from build123d import *

# Parameters (mm, degrees)
SKETCH1_W           = 216
SKETCH1_H           = 166
SKETCH1_W_2         = 40
SKETCH1_H_2         = 3
SKETCH1_W_3         = 3
SKETCH1_H_3         = 30
BOSS_EXTRUDE1_DEPTH = 3


with BuildPart() as part:
    # Sketch1 → Boss-Extrude1 (new body)
    with BuildSketch(Plane.XY):
        Rectangle(SKETCH1_W, SKETCH1_H)
        with Locations((-80, 76.5)):
            Rectangle(SKETCH1_W_2, SKETCH1_H_2, mode=Mode.SUBTRACT)
        with Locations((80, 76.5)):
            Rectangle(SKETCH1_W_2, SKETCH1_H_2, mode=Mode.SUBTRACT)
        with Locations((101.5, 30)):
            Rectangle(SKETCH1_W_3, SKETCH1_H_3, mode=Mode.SUBTRACT)
        with Locations((80, -76.5)):
            Rectangle(SKETCH1_W_2, SKETCH1_H_2, mode=Mode.SUBTRACT)
        with Locations((-101.5, 30)):
            Rectangle(SKETCH1_W_3, SKETCH1_H_3, mode=Mode.SUBTRACT)
        with Locations((0, 76.5)):
            Rectangle(SKETCH1_W_2, SKETCH1_H_2, mode=Mode.SUBTRACT)
        with Locations((101.5, -30)):
            Rectangle(SKETCH1_W_3, SKETCH1_H_3, mode=Mode.SUBTRACT)
        with Locations((0, -76.5)):
            Rectangle(SKETCH1_W_2, SKETCH1_H_2, mode=Mode.SUBTRACT)
        with Locations((-80, -76.5)):
            Rectangle(SKETCH1_W_2, SKETCH1_H_2, mode=Mode.SUBTRACT)
        with Locations((-101.5, -30)):
            Rectangle(SKETCH1_W_3, SKETCH1_H_3, mode=Mode.SUBTRACT)
    extrude(amount=BOSS_EXTRUDE1_DEPTH)


solid = part.part
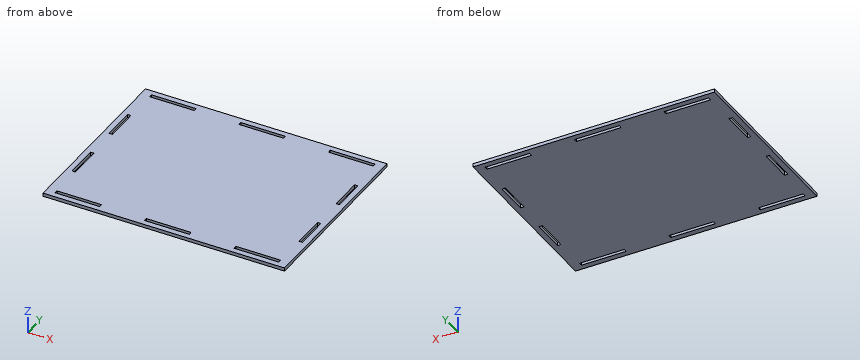
Can you work these out from the model? Positions are in its coordinate system, mm. Round coordinates to 2 decimals unless told otherwise and drop trailing zeros. Loops run counter-clockwise (first coordinate to the right, second up) from the corner with the lowest first, then second, coordinate; pieces in that order, holes last. Notation, with made-up numbers: (51, -24.5) - (60, -24.5) arc R22 ccw to (60, -16.5) - close; hole circle Ø6 at (-30, -23.75). An arc over 180 degrees is marked (long way). Write item = value, one per line. Start each with the question number.
(1) If we section it at C-C (z = 1.9): Give the number of separate pieces and of enclosed holes in the cut face, and give its area (3 significant figures).
(2) If we section it at A-A (y = 24.5): Please give me the cut outline in (x, z), and give its area (3 significant figures).
(3) If we section it at B-B (x = -9): Please give me the cut outline in (y, z).
(4) If I drill on probe 1 along X at (y, z) = (-38, 2.5); probe 2 along Y at (x, z) = (-75, 2.85), over which ranges is the centre line in solid material (lowest first)? Write a range as [from, to].
Ans:
q1.separate_pieces = 1
q1.enclosed_holes = 10
q1.area = 34,800 mm²
q2.outline = (-108, 0) - (-103, 0) - (-103, 3) - (-108, 3) - close; (-100, 0) - (100, 0) - (100, 3) - (-100, 3) - close; (103, 0) - (108, 0) - (108, 3) - (103, 3) - close
q2.area = 630 mm²
q3.outline = (-83, 0) - (-78, 0) - (-78, 3) - (-83, 3) - close; (-75, 0) - (75, 0) - (75, 3) - (-75, 3) - close; (78, 0) - (83, 0) - (83, 3) - (78, 3) - close
q4.probe_1 = [-108, -103], [-100, 100], [103, 108]
q4.probe_2 = [-83, -78], [-75, 75], [78, 83]
